Answer from the drawing. Dimensions are ordinates in mm from the lowest x, y and z of the part. A direction names the side the tool comes from. Round coordinates to 2 decimals unless told otherwise and drop trailing zeros. Loops run counter-clockwise (first coordinate to the right, second up) from the corner with the lowest first, then second, coordinate; pieces in that order, holes last. Notation, with made-up numbers: M 67,19.25 L 83,19.25 A15 ccw 83,34.25 Z; hole C 54.5,84 d4. An arc over 180 degrees is marked long. One line per item, written item: value.
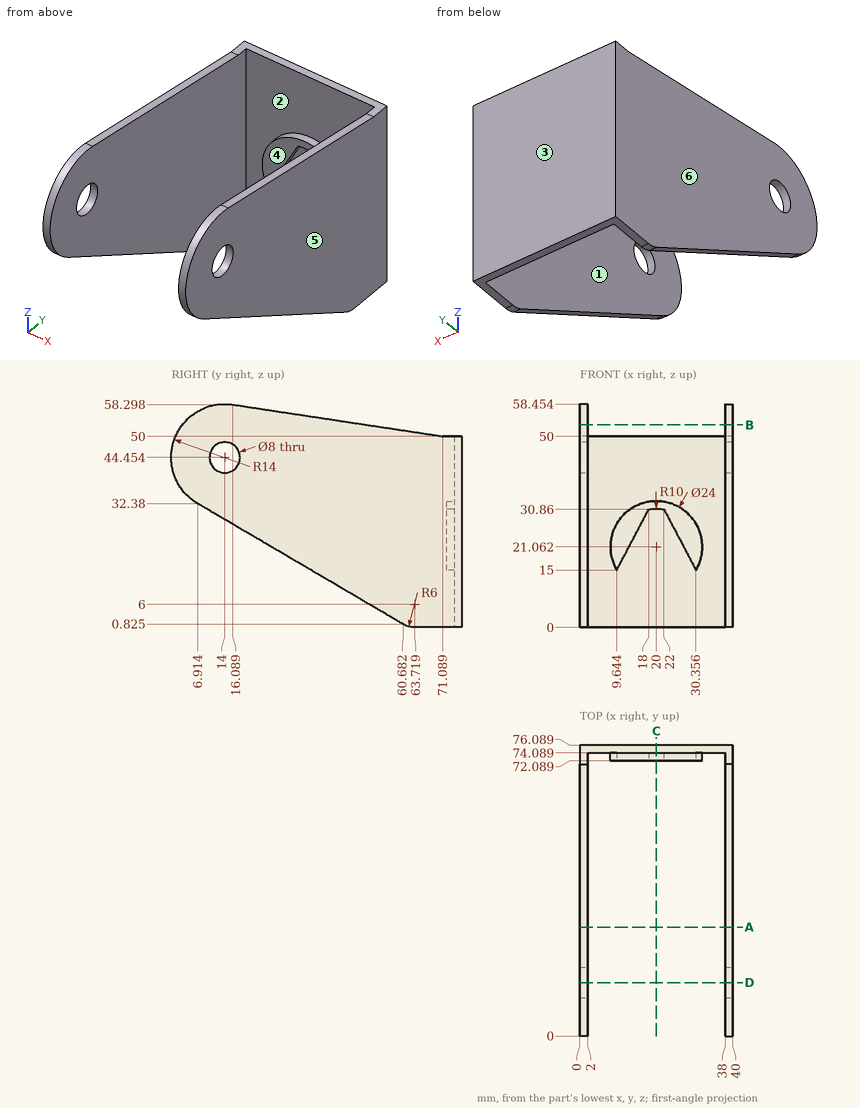
1) Each of these flat-tipped pins is pushed along its axis until it touches: pin 1 (20 mm diameter, centred on x = 16, z = 23, fed in from -Y); pin 2 (1.5 mm diameter, centred on x = 22, y = 73, fed in from +Z); pin 3 (11 mm diameter, centred on x = 19, z = 16.5, fed in from -Y). Where does it stop, or does it pass through?
Check values:
pin 1: y = 72.09
pin 2: z = 33
pin 3: y = 74.09
2) Find section C-C (x = 20). Give the vertices of the cut face in (y, z).
Check values:
outline: M 72.09,31.06 L 74.09,31.06 L 74.09,0 L 76.09,0 L 76.09,50 L 74.09,50 L 74.09,33.06 L 72.09,33.06 Z
3) Find the intervals of material crossed by probe 1 along X at (y, z) = (53, 8); probe 2 along Y at (x, z) = (37.5, 14.5); probe 3 along Y at (x, z) = (31, 18), in increasing order. Write a range as from..to.
Check values:
probe 1: 0..2, 38..40
probe 2: 74.09..76.09
probe 3: 72.09..76.09
4) For the marked faces 1 and 2, determine the directions among +Z, -Z, +X, -X, +Y, -Y from which every point of the face is accessible in a straight line to the end or side of a thin tool.
Check values:
face 1: +Z, -Z, -Y
face 2: -Y
5) Find section B-B (z = 53). Give the vertices of the cut face in (x, y), then the cut area to 3 significant figures.
Check values:
outline: M 0,2.91 L 2,2.91 L 2,51.2 L 0,51.2 Z; M 38,2.91 L 40,2.91 L 40,51.2 L 38,51.2 Z
area: 193 mm2
6) Find section A-A (y = 28.5). Give the vertices of the cut face in (x, z) (1 decimal), then the cut area to 3 significant figures.
Check values:
outline: M 0,19.7 L 2,19.7 L 2,56.4 L 0,56.4 Z; M 38,19.7 L 40,19.7 L 40,56.4 L 38,56.4 Z
area: 147 mm2
7) Find section D-D (y = 14). Give the vertices of the cut face in (x, z) (1 decimal).
Check values:
outline: M 0,28.2 L 2,28.2 L 2,40.5 L 0,40.5 Z; M 0,48.5 L 2,48.5 L 2,58.5 L 0,58.5 Z; M 38,28.2 L 40,28.2 L 40,40.5 L 38,40.5 Z; M 38,48.5 L 40,48.5 L 40,58.5 L 38,58.5 Z
8) The mould has two halves that part along X. Classify the marked faces 3, 4, 5 and 6: +X half, -X half, draft (parallel to the pull), parting line (faces both ways), or undercut.
Check values:
face 3: draft
face 4: undercut
face 5: +X half
face 6: -X half
